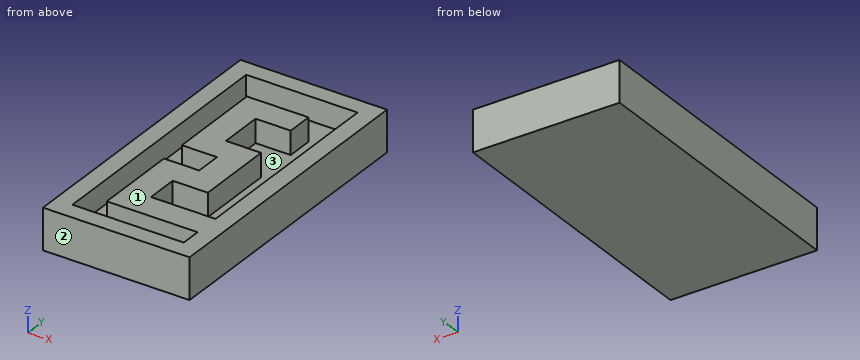
```python
from build123d import *

# Parameters (mm, degrees)
F0_W     = 5
F0_H     = 10
F1_DEPTH = 1.4
F2_T     = -0.6
F4_DEPTH = 0.8


with BuildPart() as f1:
    # F0 (on Top) → F1 (new body)
    with BuildSketch(Plane.XY):
        with Locations((4.9427011982, 1.6260683693)):
            Rectangle(F0_W, F0_H)
    extrude(amount=F1_DEPTH)

    # F2
    f2_openings = [f1.faces().sort_by_distance(p)[0] for p in [
        (4.942701, 1.626068, 1.4),
    ]]
    offset(amount=F2_T, openings=f2_openings)

    # F3 (on face) → F4 (join)
    with BuildSketch(Plane.XY.offset(0.6)):
        Polygon((6.8427011982, -2.0739316307), (6.8427011982, -1.1739316307), (4.6427011982, -1.1739316307), (4.6427011982, -0.0739316307), (5.8427011982, -0.0739316307), (5.8427011982, 2.6260683693), (4.6427011982, 2.6260683693), (4.6427011982, 4.1260683693), (5.8427011982, 4.1260683693), (5.8427011982, 5.0260683693), (3.7427011982, 5.0260683693), (3.7427011982, 1.7260683693), (4.9427011982, 1.7260683693), (4.9427011982, 0.8260683693), (3.7427011982, 0.8260683693), (3.7427011982, -2.0739316307), align=None)
    extrude(amount=F4_DEPTH)


solid = f1.part
```
CAD build for the part. Positions are in the model's coordinates, mm. Face numbers are marked on the shaded views. Round coordinates to 2 decimals unless told otherwise and drop trailing zeros. Write each loop counter-clockwise with the first axis right and the second up, starting at its lowest first coordinate (ties: lowest second). Pieces come first, ordered by that corner, then holes. Notation, with made-up numbers: (-34.75, 78) - (16.25, 78) arc R17 cw to (16.25, 83) - close; hole circle Ø1 at (37.25, 64). An arc over 180 degrees is marked (long way). Write item = value, one per line. Start each with the question number.
Q1. Band-saw the part on C-C (x = 6.7). Give the cut face in (y, z), then the cut area to 3 significant figures.
Q2. Mould opens along Y. For the marked faces 1, 2 and 3 say: pulls with the +Y half, pulls with the -Y half, needs draft (parallel to the pull), parting line crosses it, or undercut.
Q3. Band-saw the part on A-A (z = 0.9). Give the cut face in (x, y).
Q4. Band-saw the part on D-D (x = 3.55). Give the cut face in (y, z), then the cut area to 3 significant figures.
Q5. Band-saw the part on B-B (y = -0.75). Give the cut face in (x, z), then the cut area to 3 significant figures.
Q6. Probe L1, parallel to Y at x = 4.2, z = 1.15; L2, parallel to X at y = -1, z = 1.25; L3, parallel to Y at x = 5.5, z = 0.95. List the from-to ranges inside material, lowest first. Write a range as from..to.
Answers below:
q1.outline = (-3.37, 0) - (6.63, 0) - (6.63, 1.4) - (6.03, 1.4) - (6.03, 0.6) - (-1.17, 0.6) - (-1.17, 1.4) - (-2.07, 1.4) - (-2.07, 0.6) - (-2.77, 0.6) - (-2.77, 1.4) - (-3.37, 1.4) - close
q1.area = 7.68 mm2
q2.face_1 = needs draft
q2.face_2 = pulls with the -Y half
q2.face_3 = undercut
q3.outline = (2.44, -3.37) - (7.44, -3.37) - (7.44, 6.63) - (2.44, 6.63) - close; hole (3.04, -2.77) - (6.84, -2.77) - (6.84, -2.07) - (3.74, -2.07) - (3.74, 0.83) - (4.94, 0.83) - (4.94, 1.73) - (3.74, 1.73) - (3.74, 5.03) - (5.84, 5.03) - (5.84, 4.13) - (4.64, 4.13) - (4.64, 2.63) - (5.84, 2.63) - (5.84, -0.07) - (4.64, -0.07) - (4.64, -1.17) - (6.84, -1.17) - (6.84, 6.03) - (3.04, 6.03) - close
q4.outline = (-3.37, 0) - (6.63, 0) - (6.63, 1.4) - (6.03, 1.4) - (6.03, 0.6) - (-2.77, 0.6) - (-2.77, 1.4) - (-3.37, 1.4) - close
q4.area = 6.96 mm2
q5.outline = (2.44, 0) - (7.44, 0) - (7.44, 1.4) - (6.84, 1.4) - (6.84, 0.6) - (4.64, 0.6) - (4.64, 1.4) - (3.74, 1.4) - (3.74, 0.6) - (3.04, 0.6) - (3.04, 1.4) - (2.44, 1.4) - close
q5.area = 4.68 mm2
q6.L1 = -3.37..-2.77, -2.07..0.83, 1.73..5.03, 6.03..6.63
q6.L2 = 2.44..3.04, 3.74..4.64, 6.84..7.44
q6.L3 = -3.37..-2.77, -2.07..-1.17, -0.07..2.63, 4.13..5.03, 6.03..6.63
